from build123d import *

# Parameters (mm, degrees)
F1_DEPTH = 20
F2_R     = 19.99999
F4_DEPTH = 30.001


# Not quite as in the source:
# - a fillet or chamfer is up to 0.001 mm smaller than in the source, because OpenCascade refuses the exact size


with BuildPart() as f1:
    # F0 (on Front) → F1 (new body, symmetric)
    with BuildSketch(Plane.XZ):
        Polygon((0, 40), (0, 0), (50, 0), (50, 10), (30, 10), (30, 30), (20, 30), (20, 40), align=None)
    extrude(amount=F1_DEPTH, both=True)

    # F2 (radius 20 in the source; OpenCascade refuses exactly that, so slightly less here)
    f2_edges = [f1.edges().sort_by_distance(p)[0] for p in [
        (50, -20, 5),
        (50, 20, 5),
    ]]
    fillet(f2_edges, radius=F2_R)

    # F3 (on face) → F4 (cut, through all)
    with BuildSketch(Plane.XY.offset(30)):
        with BuildLine():
            Line((30, -10), (30, 10))
            ThreePointArc((30, 10), (22.9289321778, 7.0710678016), (20, -2.91e-08))
            ThreePointArc((20, -2.91e-08), (22.9289321984, -7.0710678222), (30, -10))
        make_face()
        with BuildLine():
            ThreePointArc((30, -10), (37.0710678119, -7.0710678119), (40, 0))
            ThreePointArc((40, 0), (37.0710678119, 7.0710678119), (30, 10))
            Line((30, 10), (30, -10))
        make_face()
    extrude(amount=-F4_DEPTH, mode=Mode.SUBTRACT)


solid = f1.part
Could you check a few things on this model? Use its own coordinates, in mm. A direction names the side the tool comes from. Give positions to 0.01 mm unless a question says otherwise; leave off trailing zeros. Loops run counter-clockwise (first coordinate to the right, second up) from the corner with the lowest first, then second, coordinate; pieces in that order, holes last. Notation, with made-up numbers: M 76,-4 L 129,-4 A29 ccw 129,25 Z; hole C -30,82.25 d1. An arc over 180 degrees is marked long. Answer as a JSON object with one key per item and string values.
Q1. Suppose I cut it at C-C, the plane z = 28.5. List the corners of the cut face in (x, y) for me.
Values found:
{"outline": "M 0,-20 L 30,-20 L 30,-10 A10 cw 30,10 L 30,20 L 0,20 Z"}
Q2. For P1, Ø10, axis at x = 28, y = 6, coming from the +Z side; P2, Ø6, axis at y = -2, z = 12.5, coming from the +X side; P3, Ø22, axis at x = 39.5, y = 1, coming from the +Z side, each with a flat end and sliding along its axis, tell me the tip position at first contact or that it passes through.
Values found:
{"P1": "stops at z = 30", "P2": "stops at x = 50", "P3": "stops at z = 10"}
Q3. Suppose I cut it at A-A, the plane y = 7. List the corners of the cut face in (x, z) for me (3 decimals).
Values found:
{"outline": "M 0,0 L 22.859,0 L 22.859,30 L 20,30 L 20,40 L 0,40 Z; M 37.141,0 L 48.735,0 L 48.735,10 L 37.141,10 Z"}
Q4. If we mould it in two halves opening along Y, with no side actions, what happens to faces 3 (the flat face through (25, 14, 30)), 4 (the flat face through (15, 20, 20)), 5 (the cylindrical face through (44.297, -13.986, 5.07))? For each: pulls with the +Y half, pulls with the -Y half, needs draft (parallel to the pull), parting line crosses it, or undercut.
Values found:
{"face 3": "needs draft", "face 4": "pulls with the +Y half", "face 5": "pulls with the -Y half"}
Q5. Suppose I cut it at D-D, the plane y = -16. List the corners of the cut face in (x, z) for me.
Values found:
{"outline": "M 0,0 L 42,0 L 42,10 L 30,10 L 30,30 L 20,30 L 20,40 L 0,40 Z"}
Q6. If I drill on probe 1 along X at (y, z) = (13.5, 16); probe 2 along Z at (x, y) = (40.5, -12); probe 3 along X at (y, z) = (-2.5, 34), over which ranges is the centre line in solid material (lowest first)? Write a range as [from, to].
Values found:
{"probe 1": "x = [0, 30]", "probe 2": "z = [0, 10]", "probe 3": "x = [0, 20]"}
Q7. For faces 1 (the flat face through (10, 0, 40)), 2 (the flat face through (20, 0, 35)), which set-ups out of +Z, -Z, +X, -X, +Y, -Y let a thin tool reach every point of the face, with its end or its side?
Values found:
{"face 1": "+Z, +X, -X, +Y, -Y", "face 2": "+Z, +X, +Y, -Y"}
Q8. Suppose I cut it at B-B, the plane x = 27. List the corners of the cut face in (y, z) for me.
Values found:
{"outline": "M -20,0 L -9.54,0 L -9.54,30 L -20,30 Z; M 9.54,0 L 20,0 L 20,30 L 9.54,30 Z"}
